```python
from build123d import *

# Parameters (mm, degrees)
F1_DEPTH = 12.7
F2_R     = 12.7
F3_DEPTH = 304.8
F4_R     = 12.7
F5_DEPTH = 5.08
F6_R     = 5.07999


# Not quite as in the source:
# - a fillet or chamfer is up to 0.001 mm smaller than in the source, because OpenCascade refuses the exact size


with BuildPart() as f1:
    # F0 (on Front) → F1 (new body)
    with BuildSketch(Plane.XZ):
        Polygon((-76.2, -43.9940905122), (76.2, -43.9940905122), (0, 87.9881810245), align=None)
    extrude(amount=F1_DEPTH)

    # F2 (on Front) → F3 (join)
    with BuildSketch(Plane.XZ):
        with Locations((0, -0.8957827414)):
            Circle(F2_R)
    extrude(amount=F3_DEPTH)

    # F4 (on face) → F5 (join)
    with BuildSketch(Plane.XZ.offset(304.8)):
        Circle(F4_R)
    extrude(amount=F5_DEPTH)

    # F6 (radius 5.08 in the source; OpenCascade refuses exactly that, so slightly less here)
    f6_edges = [f1.edges().sort_by_distance(p)[0] for p in [
        (-12.7, -309.88, 0),
    ]]
    fillet(f6_edges, radius=F6_R)


solid = f1.part
```
Design review of the part built by this model. Coordinates are the model's own, in mm. A direction names the side the tool comes from. Give positions to 0.01 mm unless a question says otherwise; leave off trailing zeros. Write each loop counter-clockwise with the first axis right and the second up, starting at its lowest first coordinate (ties: lowest second). Pieces come first, ordered by that corner, then holes. Notation, with made-up numbers: (-23, 84.25) -> (1, 84.25) arc R28 cw to (1, 117.25) -> close; hole circle Ø10 at (5.25, 59.5). An arc over 180 degrees is marked (long way). Answer in a Markdown table with one row per item.
(1) Clearance check with flat-ended pins moving along their axes: pin 1 (8 mm diameter, centred on x = 1, y = -236, fed in from +Z); pin 2 (14.5 mm diameter, centred on x = 5, z = 7.5, fed in from +Y); pin 3 (10 mm diameter, centred on x = -15.5, z = 63, fed in from -Y); pin 4 (2 mm diameter, centred on x = 14, y = -149.5, fed in from +Z). State where each tip first meets the part, or that it passes through.
Results:
| item | result |
|---|---|
| pin 1 | z = 11.8 |
| pin 2 | y = 0 |
| pin 3 | y = -12.7 |
| pin 4 | through |
(2) Consider section B-B (y = -247.5). State the section outline as (x, z) points.
Results:
| item | result |
|---|---|
| outline | circle Ø25.4 at (0, -0.9) |
(3) Consider section C-C (x = 44). State the section outline as (y, z) points.
Results:
| item | result |
|---|---|
| outline | (-12.7, -43.99) -> (0, -43.99) -> (0, 11.78) -> (-12.7, 11.78) -> close |
(4) Consider section A-A (x = 23). State the section outline as (y, z) points, then the cut area to 3 significant figures.
Results:
| item | result |
|---|---|
| outline | (-12.7, -43.99) -> (0, -43.99) -> (0, 48.15) -> (-12.7, 48.15) -> close |
| area | 1,170 mm2 |
(5) Mouldability with a two-part tool opening along Y and no side actions: class faces 1 (the flat face through (-1, 0, 8)), 2 (the flat face through (-1, -6, -43.994)), 3 (the cylindrical face through (-10.08, -156.71, -8.62)) as +Y half, -Y half, draft (parallel to the pull), parting line (faces both ways), or undercut.
Results:
| item | result |
|---|---|
| face 1 | +Y half |
| face 2 | draft |
| face 3 | undercut |
(6) For faces 4 (the flat face through (-37.567, -6.261, 22.921)), 5 (the flat face through (0, -304.8, -13)), 6 (the flat face through (0, -304.8, 12)), list the 3-axis set-ups (+Z, -Z, +X, -X, +Y, -Y) from which the entire face can be reached by the end or side of a thin tool; tool diameter is ignored.
Results:
| item | result |
|---|---|
| face 4 | +Z, -X, +Y, -Y |
| face 5 | -Z, -Y |
| face 6 | +Z |
(7) To check wall thickness, follow probe 1 along Z at (x, y) = (1, -78.5); probe 2 along Y at (x, z) = (31.5, 30.5); probe 3 along X at (y, z) = (-175.5, -6.5). State the ranges of each line that lie inside material, in increasing order.
Results:
| item | result |
|---|---|
| probe 1 | -13.56 to 11.76 |
| probe 2 | -12.7 to 0 |
| probe 3 | -11.4 to 11.4 |
